```python
from build123d import *

# Parameters (mm, degrees)
SZKIC1_W                    = 40
SZKIC1_H                    = 40
DODANIE_WYCI_GNI_CIE1_DEPTH = 13
OTW_R_POD_RUB_M51_D         = 5.5
SZKIC4_R                    = 6.05
WYTNIJ_WYCI_GNI_CIE1_DEPTH  = 32.128764833
WYTNIJ_WYCI_GNI_CIE2_START  = -6
SZKIC5_R                    = 2.75
WYTNIJ_WYCI_GNI_CIE2_DEPTH  = 6
SZYK_KO_OWY1_COUNT          = 4
ZAOKR_GLENIE1_R             = 5
ZAOKR_GLENIE2_R             = 3
SFAZOWANIE2_SIZE            = 1
SFAZOWANIE3_SIZE            = 0.6
SFAZOWANIE4_SIZE            = 0.5


with BuildPart() as part:
    # Szkic1 → Dodanie-wyciągnięcie1 (new body)
    with BuildSketch(Plane.XY):
        Rectangle(SZKIC1_W, SZKIC1_H)
    extrude(amount=DODANIE_WYCI_GNI_CIE1_DEPTH)

    # Otwór pod śrubę M51 (through all)
    with Locations(Plane.XY.offset(13)):
        with Locations((-14, 14), (14, 14), (14, -14), (-14, -14)):
            Hole(OTW_R_POD_RUB_M51_D / 2)

    # Szkic4 → Wytnij-wyciągnięcie1 (cut, through all)
    with BuildSketch(Plane.XY.offset(13)):
        Circle(SZKIC4_R)
        with BuildLine():
            Line((-10, 0.75), (10, 0.75))
            ThreePointArc((10, 0.75), (10.75, 0), (10, -0.75))
            Line((10, -0.75), (-10, -0.75))
            ThreePointArc((-10, -0.75), (-10.75, 0), (-10, 0.75))
        make_face()
    extrude(amount=-WYTNIJ_WYCI_GNI_CIE1_DEPTH, mode=Mode.SUBTRACT)

    # Szkic5 → Wytnij-wyciągnięcie2 (cut)
    with BuildSketch(Plane.XY.offset(13).offset(WYTNIJ_WYCI_GNI_CIE2_START)):
        with BuildLine():
            Line((6.5, 20), (6.5, 10.087120501))
            ThreePointArc((6.5, 10.087120501), (8.485281374, 8.485281374), (10.087120501, 6.5))
            Line((10.087120501, 6.5), (20, 6.5))
            Line((20, 6.5), (20, 20))
            Line((20, 20), (6.5, 20))
        make_face()
        with Locations((14, 14)):
            Circle(SZKIC5_R, mode=Mode.SUBTRACT)
    wytnij_wyci_gni_cie2 = extrude(amount=WYTNIJ_WYCI_GNI_CIE2_DEPTH, mode=Mode.SUBTRACT)

    # Szyk kołowy1: Wytnij-wyciągnięcie2 ×4 about axis
    szyk_ko_owy1_axis = Axis((0, 0, 0), (0, 0, 1))
    for i in range(1, SZYK_KO_OWY1_COUNT):
        add(wytnij_wyci_gni_cie2.rotate(szyk_ko_owy1_axis, i * 360 / SZYK_KO_OWY1_COUNT), mode=Mode.SUBTRACT)

    # Zaokrąglenie1
    zaokr_glenie1_edges = [part.edges().sort_by_distance(p)[0] for p in [
        (20, 20, 3.5),
        (20, -20, 3.5),
        (-20, -20, 3.5),
        (-20, 20, 3.5),
    ]]
    fillet(zaokr_glenie1_edges, radius=ZAOKR_GLENIE1_R)

    # Zaokrąglenie2
    zaokr_glenie2_edges = [part.edges().sort_by_distance(p)[0] for p in [
        (-10.087120501, -6.5, 10),
        (-6.5, -10.087120501, 10),
        (-6.5, -20, 10),
        (-20, -6.5, 10),
        (-6.5, 10.087120501, 10),
        (-10.087120501, 6.5, 10),
        (-20, 6.5, 10),
        (-6.5, 20, 10),
        (10.087120501, 6.5, 10),
        (6.5, 10.087120501, 10),
        (6.5, 20, 10),
        (20, 6.5, 10),
        (6.5, -10.087120501, 10),
        (10.087120501, -6.5, 10),
        (20, -6.5, 10),
        (6.5, -20, 10),
    ]]
    fillet(zaokr_glenie2_edges, radius=ZAOKR_GLENIE2_R)

    # Sfazowanie2
    sfazowanie2_edges = [part.edges().sort_by_distance(p)[0] for p in [
        (-9.25, -20, 7),
        (-20, 9.25, 7),
        (-20, 0, 0),
        (-20, -9.25, 7),
        (20, 0, 0),
        (0, -20, 0),
        (0, 20, 0),
        (18.535533906, 18.535533906, 0),
        (18.535533906, -18.535533906, 0),
        (-18.535533906, -18.535533906, 0),
        (-18.535533906, 18.535533906, 0),
        (-9.25, 20, 7),
        (-18.535533906, 18.535533906, 7),
        (9.25, -20, 7),
        (-18.535533906, -18.535533906, 7),
        (20, 9.25, 7),
        (18.535533906, -18.535533906, 7),
        (18.535533906, 18.535533906, 7),
        (9.25, 20, 7),
        (20, -9.25, 7),
    ]]
    chamfer(sfazowanie2_edges, length=SFAZOWANIE2_SIZE)

    # Sfazowanie3
    sfazowanie3_edges = [part.edges().sort_by_distance(p)[0] for p in [
        (-11.25, -14, 7),
        (-11.25, 14, 7),
        (-11.25, -14, 0),
        (16.75, -14, 0),
        (16.75, 14, 0),
        (-11.25, 14, 0),
        (16.75, 14, 7),
        (16.75, -14, 7),
    ]]
    chamfer(sfazowanie3_edges, length=SFAZOWANIE3_SIZE)

    # Szkic6 → Wycięcie-obrót1 (revolve, cut)
    with BuildSketch(Plane(origin=(0, 0, 0), x_dir=(0, 0, -1), z_dir=(1, 0, 0))):
        Polygon((-13, 9.1), (-11.4, 9.1), (-11.4, 7.525), (0, 7.525), (0, 0), (-13, 0), align=None)
    revolve(axis=Axis((0, 0, 0), (0, 0, -1)), mode=Mode.SUBTRACT)

    # Sfazowanie4
    sfazowanie4_edges = [part.edges().sort_by_distance(p)[0] for p in [
        (0, -7.525, 11.4),
        (0, -7.525, 0),
        (0, 7.525, 11.4),
        (0, 7.525, 0),
    ]]
    chamfer(sfazowanie4_edges, length=SFAZOWANIE4_SIZE)


solid = part.part
```
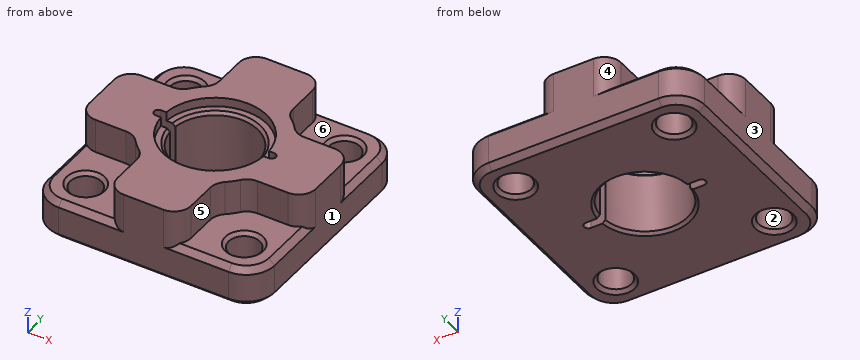
Geometry check sheet. Reference: the model listing, model coordinates, mm. Face numbers are marked on the shaded views. A direction names the side the tool comes from. Round coordinates to 2 decimals unless told otherwise and drop trailing zeros. Order: outer loops, then holes, each group sorted by start corner. A loop starts at its lowest first (then second) coordinate and runs counter-clockwise, first axis right, second up. Notation, with made-up numbers: (47.25, 51.5) - (61.25, 51.5) arc R13 ccw to (61.25, 61.5) - close; hole circle Ø3 at (-5, 57.25). An arc over 180 degrees is marked (long way). Use a Markdown table: item, result. Add a question column.
1) Set-up check for the marked faces 4, 5 and 6: record each of +Z, -Z, +X, -X, +Y, -Y from which the full face is reachable in a straight line by a thin tool's end or side.
2) Gauge pin test, flat ends, axial feed: P1, Ø2.5, axis at y = -15.5, z = 9, coming from the +X side; P2, Ø3, axis at x = 8.5, y = 15, coming from the +Z side; P3, Ø6.5, axis at x = 4, y = -5.5, coming from the +Z side; P4, Ø4, axis at y = -7.5, z = 9, coming from the -X side. Record the tip position at first contact, or that the pin passes through.
3) Mould release check, pull along X, two halves, no side actions. Record for the marked faces 1, 2 and 3: released by +X, released by -X, zero draft, split by the parting line, or undercut.
4) Section check D-D (y = 0). Record the cut outline in (x, z), then the cut area to 4 significant figures.
5) Thickness scan on line 1 along Y through (x, z) = (-14, 3); line 2 along Y through (x, z) = (8.5, 1.75). Record the ranges inside material, lowest first.
6) Section check A-A (x = -14). Record the cut outline in (y, z).
7) Section check B-B (z = 4). Record the cut outline in (x, y) (3 decimals).
Established:
| question | item | result |
|---|---|---|
| 1 | face 4 | +Z, -X, +Y |
| 1 | face 5 | +Z, +X, -Y |
| 1 | face 6 | +Z, +X, +Y |
| 2 | P1 | x = 6.5 |
| 2 | P2 | z = 7 |
| 2 | P3 | z = 13 |
| 2 | P4 | x = -19.24 |
| 3 | face 1 | released by +X |
| 3 | face 2 | undercut |
| 3 | face 3 | released by -X |
| 4 | outline | (-20, 1) - (-19, 0) - (-10.75, 0) - (-10.75, 13) - (-20, 13) - close; (10.75, 0) - (19, 0) - (20, 1) - (20, 13) - (10.75, 13) - close |
| 4 | area | 239.5 mm2 |
| 5 | line 1 | -20 to -16.75, -11.25 to 11.25, 16.75 to 20 |
| 5 | line 2 | -20 to -0.75, 0.75 to 20 |
| 6 | outline | (-20, 1) - (-19, 0) - (-17.35, 0) - (-16.75, 0.6) - (-16.75, 6.4) - (-17.35, 7) - (-19, 7) - (-20, 6) - close; (-11.25, 0.6) - (-10.65, 0) - (10.65, 0) - (11.25, 0.6) - (11.25, 6.4) - (10.65, 7) - (6.5, 7) - (6.5, 13) - (-6.5, 13) - (-6.5, 7) - (-10.65, 7) - (-11.25, 6.4) - close; (16.75, 0.6) - (17.35, 0) - (19, 0) - (20, 1) - (20, 6) - (19, 7) - (17.35, 7) - (16.75, 6.4) - close |
| 7 | outline | (-20, -15) arc R5 ccw to (-15, -20) - (15, -20) arc R5 ccw to (20, -15) - (20, 15) arc R5 ccw to (15, 20) - (-15, 20) arc R5 ccw to (-20, 15) - close; hole circle Ø5.5 at (-14, -14); hole circle Ø5.5 at (-14, 14); hole (-10, -0.75) - (-7.488, -0.75) arc R7.525 ccw to (7.488, -0.75) - (10, -0.75) arc R0.75 ccw to (10, 0.75) - (7.488, 0.75) arc R7.525 ccw to (-7.488, 0.75) - (-10, 0.75) arc R0.75 ccw to start; hole circle Ø5.5 at (14, -14); hole circle Ø5.5 at (14, 14) |
